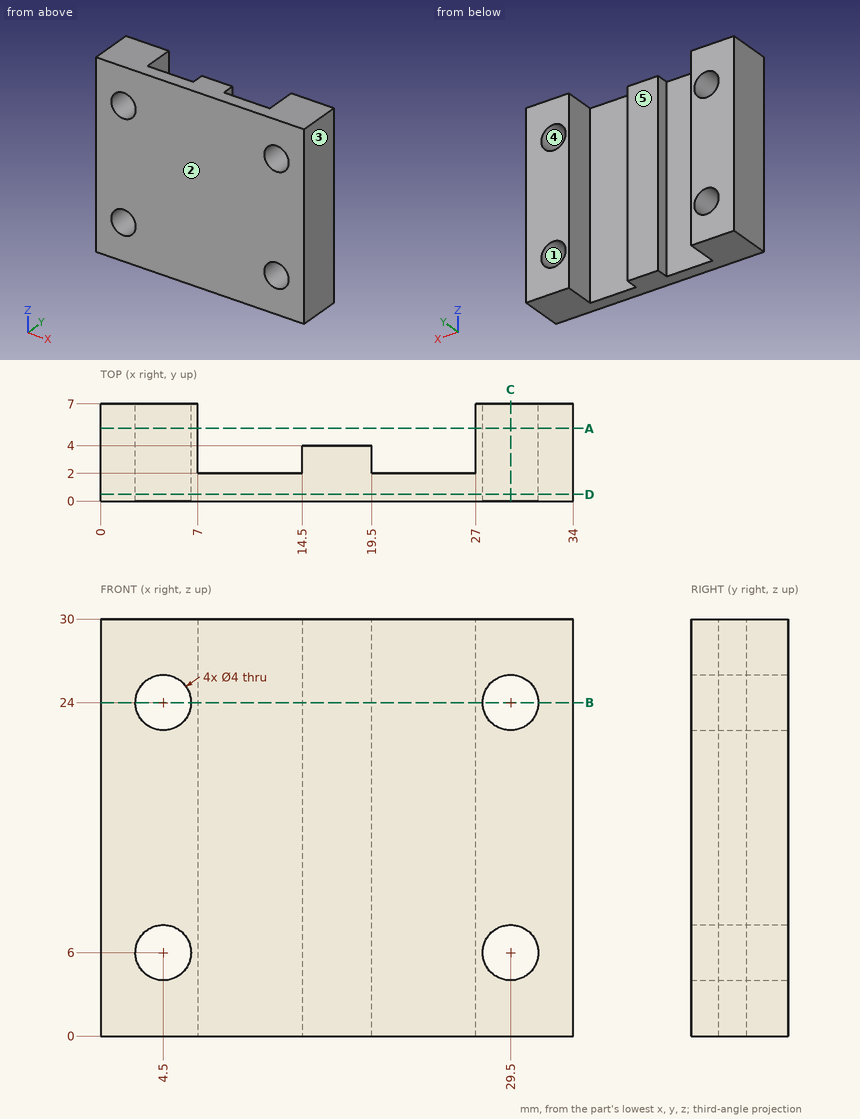
Could you check a few things on this drawing? It's one solid part, dimensions in mm from its lowest x, y, z. A direction names the side the tool comes from. Round coordinates to 2 decimals unless told otherwise and drop trailing zeros. Order: outer loops, then holes, each group sorted by start corner. A loop starts at its lowest first (then second) coordinate and runs counter-clockwise, first axis right, second up.
(1) Imagine slicing it at A-A (y = 5.25). Write out the boundary of the cut face in (x, z).
Response values:
outline: (0, 0) - (7, 0) - (7, 30) - (0, 30) - close; (27, 0) - (34, 0) - (34, 30) - (27, 30) - close; hole circle Ø4 at (4.5, 6); hole circle Ø4 at (4.5, 24); hole circle Ø4 at (29.5, 6); hole circle Ø4 at (29.5, 24)
(2) Imagine slicing it at D-D (y = 0.5). Write out the boundary of the cut face in (x, z).
Response values:
outline: (0, 0) - (34, 0) - (34, 30) - (0, 30) - close; hole circle Ø4 at (4.5, 6); hole circle Ø4 at (4.5, 24); hole circle Ø4 at (29.5, 6); hole circle Ø4 at (29.5, 24)
(3) Imagine slicing it at C-C (x = 29.5). Write out the boundary of the cut face in (y, z), plus the area to 3 significant figures.
Response values:
outline: (0, 0) - (7, 0) - (7, 4) - (0, 4) - close; (0, 8) - (7, 8) - (7, 22) - (0, 22) - close; (0, 26) - (7, 26) - (7, 30) - (0, 30) - close
area: 154 mm2
(4) Which directions (+Z, -Z, +X, -X, +Y, -Y) give clear straight access to the entire face, cutting with the end or side of a thin tool? Please do the marked faces 4 and 5.
Response values:
face 4: +Y, -Y
face 5: +Z, -Z, +Y
(5) If we mould it in two halves opening along X, with no side actions, what happens to the marked faces 1, 2 and 3? For each: released by +X, released by -X, zero draft, split by the parting line, or undercut.
Response values:
face 1: undercut
face 2: zero draft
face 3: released by +X
(6) Please list where these lines run through material, in increasing order: line 1 along Z through (x, y) = (29.5, 5.25); line 2 along X through (y, z) = (5, 6); line 3 along X through (y, z) = (2.75, 16.75).
Response values:
line 1: z = 0 to 4, 8 to 22, 26 to 30
line 2: x = 0 to 2.5, 6.5 to 7, 27 to 27.5, 31.5 to 34
line 3: x = 0 to 7, 14.5 to 19.5, 27 to 34
(7) I'm going to push flat-ended pins straight in: pin 1 (10 mm diameter, centred on x = 13, z = 6, fed in from +Y); pin 2 (4 mm diameter, centred on x = 22.5, z = 19.5, fed in from +Y). Where does each tip first touch, or does it pass through?
Response values:
pin 1: stops at y = 4
pin 2: stops at y = 2
(8) Imagine slicing it at B-B (z = 24). Write out the boundary of the cut face in (x, y), plus the area to 3 significant figures.
Response values:
outline: (0, 0) - (2.5, 0) - (2.5, 7) - (0, 7) - close; (6.5, 0) - (27.5, 0) - (27.5, 7) - (27, 7) - (27, 2) - (19.5, 2) - (19.5, 4) - (14.5, 4) - (14.5, 2) - (7, 2) - (7, 7) - (6.5, 7) - close; (31.5, 0) - (34, 0) - (34, 7) - (31.5, 7) - close
area: 92.0 mm2
